Work out the finished part from the listing and answer in its coordinate system (mm). A direction names the side the tool comes from. Coordinates: 2 decimals unless noted, no trailing zeros. Loops run counter-clockwise (first coordinate to the right, second up) from the corner with the lowest first, then second, coordinate; pieces in that order, holes last. Notation, with made-up numbers: M -29,78.5 L -14,78.5 A23 ccw -14,117.5 Z; hole C 84,-8.75 d7. An arc over 180 degrees is marked long. Write each question's results on one line, items separated by ' | '.
```python
from build123d import *

# Parameters (mm, degrees)
SKETCH1_R                = 7
BOSS_EXTRUDE1_DEPTH      = 12
SKETCH2_R                = 24
BOSS_EXTRUDE2_DEPTH      = 48
BOSS_EXTRUDE3_DEPTH      = 12
SKETCH4_R                = 15
BOSS_EXTRUDE4_DEPTH      = 26
SKETCH5_R                = 12
BOSS_EXTRUDE5_DEPTH      = 26
BOSS_EXTRUDE6_DEPTH      = 24
BOSS_EXTRUDE6_DEPTH_BACK = 24
FILLET2_R                = 6
BOSS_EXTRUDE8_DEPTH      = 12
BOSS_EXTRUDE8_DEPTH_BACK = 12


with BuildPart() as part:
    # Sketch1 → Boss-Extrude1 (new body)
    with BuildSketch(Plane(origin=(0, 0, 0), x_dir=(0, 0, -1), z_dir=(1, 0, 0))):
        with BuildLine():
            Line((-59.995604766, 5.505634955), (-40.05091289, -71.438574032))
            ThreePointArc((-40.05091289, -71.438574032), (-33.642720476, -81.157532712), (-22.626759324, -84.92206293))
            Line((-22.626759324, -84.92206293), (22.246130308, -84.92206293))
            ThreePointArc((22.246130308, -84.92206293), (33.289539949, -81.136249628), (39.687584355, -71.371296652))
            Line((39.687584355, -71.371296652), (59.315693821, 5.572912335))
            ThreePointArc((59.315693821, 5.572912335), (56.088426472, 21.065555698), (41.874239774, 28.022146056))
            Line((41.874239774, 28.022146056), (-42.571451201, 28.022146056))
            ThreePointArc((-42.571451201, 28.022146056), (-56.806920983, 21.038107208), (-59.995604766, 5.505634955))
        make_face()
        with Locations((-42, 10.022146056)):
            Circle(SKETCH1_R, mode=Mode.SUBTRACT)
        with Locations((-22.626759324, -66.92206293)):
            Circle(SKETCH1_R, mode=Mode.SUBTRACT)
        with Locations(Location((42, 10.022146056, 0), (0, 0, 180))):
            Circle(SKETCH1_R, mode=Mode.SUBTRACT)
        with Locations(Location((22.626759324, -66.92206293, 0), (0, 0, 180))):
            Circle(SKETCH1_R, mode=Mode.SUBTRACT)
    extrude(amount=BOSS_EXTRUDE1_DEPTH)



with BuildPart() as body_2:
    # Sketch2 → Boss-Extrude2 (new body)
    with BuildSketch(Plane(origin=(36, 0, 0), x_dir=(0, 0, -1), z_dir=(1, 0, 0))):
        with Locations((0, 78.07793707)):
            Circle(SKETCH2_R)
    extrude(amount=BOSS_EXTRUDE2_DEPTH)

    # Sketch3 → Boss-Extrude3 (add)
    with BuildSketch(Plane(origin=(84, 0, 0), x_dir=(0, 0, -1), z_dir=(1, 0, 0))):
        with BuildLine():
            Line((-24, 78.07793707), (24, 78.07793707))
            ThreePointArc((24, 78.07793707), (0, 54.07793707), (-24, 78.07793707))
        make_face()
    extrude(amount=BOSS_EXTRUDE3_DEPTH)

    # Sketch4 → Boss-Extrude4 (add)
    with BuildSketch(Plane(origin=(96, 0, 0), x_dir=(0, 0, -1), z_dir=(1, 0, 0))):
        with Locations((0, 78.07793707)):
            Circle(SKETCH4_R)
    extrude(amount=BOSS_EXTRUDE4_DEPTH)

    # Sketch5 → Boss-Extrude5 (add)
    with BuildSketch(Plane.ZY.offset(-36)):
        with Locations(Location((0, 78.07793707, 0), (0, 0, 180))):
            Circle(SKETCH5_R)
    extrude(amount=BOSS_EXTRUDE5_DEPTH)


with BuildPart() as part_1:
    add(part.part)

    add(body_2.part)  # Boss-Extrude6 merges body 2
    # Sketch6 → Boss-Extrude6 (add, two sides: drawn at the far end of the back side and taken through both)
    with BuildSketch(Plane.XY.offset(-BOSS_EXTRUDE6_DEPTH_BACK)):
        Polygon((12, 28.022146056), (48, 28.022146056), (48, 77.929166674), (60, 77.929166674), (60, 16.022146056), (12, 16.022146056), align=None)
    extrude(amount=BOSS_EXTRUDE6_DEPTH + BOSS_EXTRUDE6_DEPTH_BACK)

    # Fillet2
    fillet2_edges = [part_1.edges().sort_by_distance(p)[0] for p in [
        (48, 28.022146056, 0),
    ]]
    fillet(fillet2_edges, radius=FILLET2_R)

    # Sketch8 → Boss-Extrude8 (add, two sides: drawn at the far end of the back side and taken through both)
    with BuildSketch(Plane.XY.offset(-BOSS_EXTRUDE8_DEPTH_BACK)):
        Polygon((96, 78.07793707), (60, 77.929166674), (60, 54.07793707), (60, 16.022146056), (12, 16.022146056), (12, -84.92206293), (96, 54.07793707), align=None)
    extrude(amount=BOSS_EXTRUDE8_DEPTH + BOSS_EXTRUDE8_DEPTH_BACK)


solid = part_1.part
```
1) Find section C-C, the plane x = 104.5. Give the vertices of the cut face in (y, z).
Check result:
outline: C 78.08,0 d30
2) Find section D-D, the plane y = 44.5. Give the vertices of the cut face in (x, z), and give its area (3 significant figures).
Check result:
outline: M 48,-24 L 60,-24 L 60,-12 L 90.21,-12 L 90.21,12 L 60,12 L 60,24 L 48,24 Z | area: 1,300 mm^2
3) Straight lines are drawn through the part: probe 1 along X at (y, z) = (-61.5, -38.5); probe 2 along Z at (x, y) = (27.5, -57.5); probe 3 along X at (y, z) = (23.5, 16.5). For each, find the intervals that lie inside material, in ascending order. Write a range as [from, to].
Check result:
probe 1: [0, 12] | probe 2: [-12, 12] | probe 3: [0, 60]
4) Find section B-B, the plane z = 0. Give the vertices of the cut face in (x, y), and give its area (3 significant figures).
Check result:
outline: M 0,-84.92 L 12,-84.92 L 96,54.08 L 96,63.08 L 122,63.08 L 122,93.08 L 96,93.08 L 96,78.08 L 84,78.08 L 84,102.08 L 36,102.08 L 36,90.08 L 10,90.08 L 10,66.08 L 36,66.08 L 36,54.08 L 48,54.08 L 48,34.02 A6 cw 42,28.02 L 0,28.02 Z | area: 10,300 mm^2
5) Which of the six approach directions +Z, -Z, +X, -X, +Y, -Y give full straight-line access (tool end or side, diameter ignored) to faces 4 (the face through (52, 34, 24)), 5 (the face through (36, 16.022, 18)), 6 (the face through (60, 41, -18)), 7 (the face through (96, 84, 0)), 8 (the face through (10, 78, 0))?
Check result:
face 4: +Z, +X, +Y, -Y | face 5: +Z, +X, -Y | face 6: -Z, +X, -Y | face 7: +Z, -Z, +Y | face 8: +Z, -Z, -X, +Y
6) For a pull along Y with two mould halves and no side action, classify faces 1 (the face through (5.916, -81.238, -33.158)), 2 (the face through (108.818, 68.951, 11.903)), 3 (the face through (5.916, -71.181, 28.182)) as released by +Y, released by -Y, zero draft, split by the parting line, or undercut.
Check result:
face 1: released by -Y | face 2: split by the parting line | face 3: undercut
7) Find section A-A, the plane y = -62.5. Give the vertices of the cut face in (x, z).
Check result:
outline: M 0,-41.95 L 12,-41.95 L 12,-28.05 L 0,-28.05 Z; M 0,-17.2 L 12,-17.2 L 12,-12 L 25.55,-12 L 25.55,12 L 12,12 L 12,17.2 L 0,17.2 Z; M 0,28.05 L 12,28.05 L 12,42.37 L 0,42.37 Z
8) Given pin 1 Ø9.5 at (y, z) = (48.5, -19.5) entering from +X; pin 2 Ø10 at (y, z) = (47.5, -17.5) entering from -X; pin 3 Ø12 at (x, z) = (40.5, -18.5) entering from -Y; pin 4 Ø8.5 at (y, z) = (10.02, 42) entering from -X, each flat-ended and moving along its own axis, determine where each tip first touches the part or whether it passes through.
Check result:
pin 1: x = 60 | pin 2: x = 48 | pin 3: y = 16.02 | pin 4: through
